Input: part model. Units: mm. Frame: model coordinates. A direction names the side the tool comes from. Give positions to 0.01 mm unless a question says otherwise; leave off trailing zeros. Write each loop counter-clockwise with the first axis right and the second up, starting at its lowest first coordinate (ties: lowest second). Pieces come first, ordered by that corner, then holes. Notation, with made-up numbers: (71.25, 89.5) - (106.25, 89.5) arc R19 ccw to (106.25, 96.5) - close; hole circle Ø11 at (8.25, -30.5). An arc over 180 degrees is marked (long way). Use a Markdown table: item, result. Add a question column.
1. Pin query (flat end, axial travel): pin 1 (1.7 mm diameter, centred on y = 4.5, z = -28.5, fed in from -X); pin 2 (5 mm diameter, centred on x = -13, z = 12, fed in from +Y); pin 3 (4 mm diameter, centred on x = -29.68, z = 0, fed in from +Y); pin 4 (2 mm diameter, centred on x = 30.5, z = -20.5, fed in from +Y). Return the tip coordinate at first contact, or that it passes through.
2. Section query A-A, the plane y = 7.75. Return loops of the section in (x, z).
3. Set-up query: faces 4 (the flat face through (17, 5.093, -30)), 5 (the cylindrical face through (-0.48, 5, -3.25)), 6 (the flat face through (-23.558, 13, -27)), 7 (the cylindrical face through (17.12, 14.422, 27.304)), 8 (the flat face through (-38.43, 9, 0)). Return all of +Z, -Z, +X, -X, +Y, -Y with unobstructed straight access to the full face (end or side cutting, diameter ignored); none if empty.
4. Section query B-B, the plane x = 26. Return loops of the section in (y, z), plus the area to 3 significant figures.
5. Section query D-D, the plane y = 13. Return loops of the section in (x, z).
6. Material intervals for probe 1 along X at (y, z) = (2.25, 0); probe 2 along X at (y, z) = (3, -6); probe 3 along Z at (x, y) = (-18.5, 6), sorted ascending.
7. Mould query, pull axis Z, two halves, no side actions, for faces 1 (the flat face through (-17, 3.505, 30)), 2 (the flat face through (-22.754, 4.31, -30.332)), 3 (the cylindrical face through (-0.48, 5.13, 3.15)). Classes: released by +Z, released by -Z, zero draft, split by the parting line, or undercut.
8. Section query C-C, the plane z = -14. Return loops of the section in (x, y) (1 decimal).
Autodesk Inventor part; units mm, degrees
ref_plane "Work Plane1" through (0, 0, 27.94) normal (1, 0, 0) x (0, 0, -1)
ref_plane "Work Plane2" through (-38.4302, 0, 0) normal (0, 0, 1) x (1, 0, 0)
ref_plane "YZ Plane" through (0, 0, 0) normal (1, 0, 0) x (0, 1, 0)
sketch "Sketch1" plane through (0, 0, 0) normal (0, 1, 0) x (-1, 0, 0)
  line L0 (38.4302, 27.94) -> (-38.4302, 27.94)
  line L1 (-38.4302, 27.94) -> (-38.4302, -27.94)
  line L2 (-38.4302, -27.94) -> (38.4302, -27.94)
  line L3 (38.4302, -27.94) -> (38.4302, 27.94)
  line L4 (53.8023, 0) -> (-53.8023, 0) construction
  line L5 (0, -39.116) -> (0, 39.116) construction
  point P0 (0, 0)
  point P1 (0, 27.94)
  point P2 (38.4302, 0)
  dimension "d0" = 76.8604
  dimension "d1" = 55.88
extrude "Extrusion1" add sketch "Sketch1" along normal blind 18.415
ref_plane "Work Plane1" through (0, 0, 27.94) normal (1, 0, 0) x (0, 0, -1)
sketch "Sketch2" plane through (0, 0, 27.94) normal (1, 0, 0) x (0, 0, -1)
  line L0 (27.94, -6.8898) -> (27.94, 29.6482) construction
  line L1 (67.056, 0) -> (-11.176, 0) construction
  circle A0 centre (14.5034, 13.1588) radius 13.0493
  circle A1 centre (41.3766, 13.1588) radius 13.0493
  line L2 (1.8034, 10.16) -> (27.2034, 10.16) construction
  point P0 (27.94, 0)
  dimension "d4" = 13.4366
  dimension "d6" = 26.0985
  dimension "d11" = 25.4
  dimension "d12" = 10.16
extrude "Extrusion2" cut sketch "Sketch2" along normal mid plane 68.961
sketch "Sketch3" plane through (-38.4302, 0, 27.94) normal (0, 0, 1) x (1, 0, 0)
  line L0 (0, 18.415) -> (76.8604, 18.415) construction
  line L1 (3.9497, 18.415) -> (3.9497, 0.1096) construction
  line L2 (3.9497, 18.415) -> (14.8717, 18.415)
  line L3 (14.8717, 18.415) -> (14.8717, 10.16)
  line L4 (14.8717, 10.16) -> (3.9497, 10.16)
  line L5 (3.9497, 10.16) -> (3.9497, 18.415)
  line L6 (27.5717, 18.415) -> (38.4302, 18.415)
  line L7 (27.5717, 10.16) -> (27.5717, 18.415)
  line L8 (-15.3721, 0) -> (92.2325, 0) construction
  line L9 (27.5717, 10.16) -> (38.4302, 10.16)
  line L10 (38.4302, -3.683) -> (38.4302, 22.098) construction
  line L11 (72.9107, 18.415) -> (61.9887, 18.415)
  line L12 (61.9887, 18.415) -> (61.9887, 10.16)
  line L13 (61.9887, 10.16) -> (72.9107, 10.16)
  line L14 (72.9107, 10.16) -> (72.9107, 18.415)
  line L15 (49.2887, 18.415) -> (38.4302, 18.415)
  line L16 (49.2887, 10.16) -> (49.2887, 18.415)
  line L17 (49.2887, 10.16) -> (38.4302, 10.16)
  point P0 (38.4302, 0)
  dimension "d13" = 10.922
  dimension "d16" = 10.16
  dimension "d17" = 12.7
extrude "Extrusion3" cut sketch "Sketch3" against normal through all
sketch "Sketch4" plane through (-34.4805, 0, 27.94) normal (1, 0, 0) x (0, 0, -1)
  line L0 (27.2034, 10.16) -> (28.6766, 10.16)
  arc A0 (27.2034, 10.16) -> (26.4472, 18.415) centre (14.5034, 13.1588) ccw
  arc A1 (29.4328, 18.415) -> (28.6766, 10.16) centre (41.3766, 13.1588) ccw
  line L1 (29.4328, 18.415) -> (26.4472, 18.415)
  line L2 (0, 18.415) -> (2.5596, 18.415)
  arc A2 (2.5596, 18.415) -> (0, 10.16) centre (14.5917, 10.16) ccw
  line L3 (0, 18.415) -> (55.88, 18.415) construction
  line L4 (0, 10.16) -> (0, 18.415)
  line L5 (0, 18.415) -> (2.5596, 18.415)
  line L6 (27.94, -3.7218) -> (27.94, 22.3306) construction
  line L7 (55.88, 18.415) -> (53.3204, 18.415)
  arc A3 (55.88, 10.16) -> (53.3204, 18.415) centre (41.2883, 10.16) ccw
  line L8 (55.88, 10.16) -> (55.88, 18.415)
  line L9 (55.88, 18.415) -> (53.3204, 18.415)
  point P0 (27.94, 0)
  point P1 (0, 0)
  dimension "d21" = 14.5917
extrude "Extrusion4" cut sketch "Sketch4" along normal up to surface (68.961 mm away)
sketch "Sketch5" plane through (-34.4805, 0, 27.94) normal (1, 0, 0) x (0, 0, -1)
  arc A0 (1.8034, 10.16) -> (27.2034, 10.16) centre (14.5034, 13.1588) ccw construction
  arc A1 (28.6766, 10.16) -> (54.0766, 10.16) centre (41.3766, 13.1588) ccw construction
  line L0 (27.2034, 10.16) -> (28.6766, 10.16)
  line L1 (22.479, 2.8306) -> (33.401, 2.8306)
  arc A2 (22.479, 2.8306) -> (27.2034, 10.16) centre (14.5034, 13.1588) ccw
  arc A3 (28.6766, 10.16) -> (33.401, 2.8306) centre (41.3766, 13.1588) ccw
  point P0 (27.94, 0)
  dimension "d24" = 10.922
extrude "Extrusion5" cut sketch "Sketch5" along normal blind 9.652
mirror "Mirror1" about plane through (0, 0, 27.94) normal (1, 0, 0) of "Extrusion5"
sketch "Sketch6" plane through (-34.4805, 0, 27.94) normal (1, 0, 0) x (0, 0, -1)
  arc A0 (1.8034, 10.16) -> (22.479, 2.8306) centre (14.5034, 13.1588) ccw construction
  line L0 (55.88, 0) -> (0, 0) construction
  line L1 (8.6614, 1.4903) -> (8.6614, 0)
  line L2 (14.5034, 13.1588) -> (14.5034, 0) construction
  line L3 (20.3454, 1.4903) -> (20.3454, 0)
  arc A1 (8.6614, 1.4903) -> (20.3454, 1.4903) centre (14.5034, 13.1588) ccw
  line L4 (8.6614, 0) -> (20.3454, 0)
  point P0 (27.94, 0)
  dimension "d27" = 5.842
extrude "Extrusion6" cut sketch "Sketch6" along normal up to surface (68.961 mm away)
ref_plane "Work Plane2" through (-38.4302, 0, 0) normal (0, 0, 1) x (1, 0, 0)
mirror "Mirror2" about plane through (-38.4302, 0, 0) normal (0, 0, 1) of "Extrusion6"
sketch "Sketch7" plane through (38.4302, 0, 27.94) normal (1, 0, 0) x (0, 0, -1)
  line L0 (0, 0) -> (0, 18.415) construction
  line L1 (0, 18.415) -> (55.88, 18.415) construction
  arc A0 (2.5596, 18.415) -> (0, 10.16) centre (14.5917, 10.16) ccw construction
  line L2 (2.5596, 18.415) -> (0, 10.16)
  line L3 (2.5596, 18.415) -> (0, 18.415)
  line L4 (0, 10.16) -> (0, 18.415)
  point P0 (27.94, 0)
extrude "Extrusion7" cut sketch "Sketch7" against normal up to surface (3.9497 mm away)
mirror "Mirror3" about plane through (-38.4302, 0, 0) normal (0, 0, 1) of "Extrusion7"
mirror "Mirror4" about plane through (0, 0, 27.94) normal (1, 0, 0) of "Extrusion7", "Mirror3"
fillet "Fillet1" radius 1.5875 4 edges at (-34.4805, 10.16, -27.0383) (-34.4805, 10.16, 27.0383) (34.4805, 10.16, -27.0383) (34.4805, 10.16, 27.0383)
sketch "Sketch9" plane through (-38.4302, 0, 27.94) normal (0, 0, 1) x (1, 0, 0)
  line L0 (27.5717, 10.16) -> (27.5717, 18.415) construction
  line L1 (14.8717, 18.415) -> (14.8717, 10.16) construction
  line L2 (0, 0) -> (76.8604, 0) construction
  line L3 (14.8717, 5.0927) -> (14.8717, 3.5052)
  line L4 (27.5717, 5.0927) -> (27.5717, 3.5052)
  line L5 (14.8717, 5.0927) -> (27.5717, 5.0927)
  line L6 (14.8717, 3.5052) -> (27.5717, 3.5052)
  point P0 (38.4302, 0)
  dimension "d33" = 3.5052
  dimension "d34" = 1.5875
  dimension "d36" = 12.7
  dimension "d37" = 12.7
extrude "Extrusion8" add sketch "Sketch9" along normal blind 3.175
mirror "Mirror5" about plane through (0, 0, 27.94) normal (1, 0, 0) of "Extrusion8"
mirror "Mirror6" about plane through (-38.4302, 0, 0) normal (0, 0, 1) of "Extrusion8", "Mirror5"
chamfer "Chamfer1" distance 1.5875 angle 45 8 edges at (-10.8585, 4.299, 31.115) (23.5585, 4.2989, 31.115) (10.8585, 4.299, 31.115) (-23.5585, 4.2989, 31.115) (-10.8585, 4.299, -31.115) (-23.5585, 4.2989, -31.115) (23.5585, 4.2989, -31.115) (10.8585, 4.299, -31.115)
sketch "Sketch10" plane through (-34.4805, 2.8306, 5.461) normal (0, 1, 0) x (1, 0, 0)
  line L0 (-19.3218, 5.461) -> (88.2828, 5.461) construction
  line L1 (34.4805, 49.022) -> (34.4805, -38.1) construction
  point P0 (34.4805, 5.461)
  point P1 (4.8006, 5.461)
  dimension "d43" = 29.6799
hole "Hole1" at (-29.6799, 2.8306, 0) direction (0, -1, 0) diameter 3.6576 end through all
mirror "Mirror7" about plane through (0, 0, 27.94) normal (1, 0, 0) of "Hole1"
properties part number "Keystone-26650-Dual-Battery-Holder[DWG-1109]" material "Thermoplastic Resin"
Result sheet:
| question | item | result |
|---|---|---|
| 1 | pin 1 | stops at x = -38.43 |
| 1 | pin 2 | passes through |
| 1 | pin 3 | stops at y = 2.83 |
| 1 | pin 4 | stops at y = 2.9 |
| 2 | outline | (-38.43, -27.94) - (38.43, -27.94) - (38.43, 27.94) - (-38.43, 27.94) - close; (-24.83, -1.56) - (24.83, -1.56) - (24.83, 1.56) - (-24.83, 1.56) - close; hole (-34.48, -25.31) - (34.48, -25.31) - (34.48, 25.31) - (-34.48, 25.31) - close |
| 3 | face 4 | -Z, +X, -X, +Y |
| 3 | face 5 | +Y |
| 3 | face 6 | +Z, -Z, +Y |
| 3 | face 7 | +Z, +X, -X, +Y |
| 3 | face 8 | +Z, -Z, -X, +Y, -Y |
| 4 | outline | (0, -27.94) - (10.16, -27.94) - (10.16, -26.14) arc R13.05 cw to (1.49, -19.28) - (0, -19.28) - close; (0, -7.59) - (1.49, -7.59) arc R13.05 cw to (2.83, -5.46) - (2.83, 5.46) arc R13.05 cw to (1.49, 7.59) - (0, 7.59) - close; (0, 19.28) - (1.49, 19.28) arc R13.05 cw to (10.16, 26.14) - (10.16, 27.94) - (0, 27.94) - close |
| 4 | area | 138 mm² |
| 5 | outline | (-38.43, -27.06) - (-34.48, -27.06) - (-34.48, 27.06) - (-38.43, 27.06) - close; (-23.56, -27.66) - (-10.86, -27.66) - (-10.86, -26.48) - (-23.56, -26.48) - close; (-23.56, 26.48) - (-10.86, 26.48) - (-10.86, 27.66) - (-23.56, 27.66) - close; (10.86, -27.66) - (23.56, -27.66) - (23.56, -26.48) - (10.86, -26.48) - close; (10.86, 26.48) - (23.56, 26.48) - (23.56, 27.66) - (10.86, 27.66) - close; (34.48, -27.06) - (38.43, -27.06) - (38.43, 27.06) - (34.48, 27.06) - close |
| 6 | probe 1 | x = -38.43 to -31.51, -27.85 to 27.85, 31.51 to 38.43 |
| 6 | probe 2 | x = -38.43 to -34.48, 34.48 to 38.43 |
| 6 | probe 3 | z = -27.94 to -24.35, -2.53 to 2.53, 24.35 to 27.94 |
| 7 | face 1 | zero draft |
| 7 | face 2 | released by -Z |
| 7 | face 3 | undercut |
| 8 | outline | (-38.4, 0) - (-34.5, 0) - (-34.5, 18.4) - (-38.4, 18.4) - close; (34.5, 0) - (38.4, 0) - (38.4, 18.4) - (34.5, 18.4) - close |
